```python
from build123d import *

# Parameters (mm, degrees)
SZKIC1_R                    = 7.5
SZKIC1_R_2                  = 3
DODANIE_WYCI_GNI_CIE1_DEPTH = 15
DODANIE_WYCI_GNI_CIE2_START = -15
SZKIC1_3_R                  = 7.5
SZKIC1_3_R_2                = 3
DODANIE_WYCI_GNI_CIE2_DEPTH = 15


with BuildPart() as part:
    # Szkic1 → Dodanie-wyciągnięcie1 (new body)
    # profile 1 of 2: a face of its own
    with BuildSketch(Plane(origin=(0, 0, 0), x_dir=(1, 0, 0), z_dir=(0, 1, 0))):
        Polygon((-5.484827557, -9.5), (5.484827557, -9.5), (10.969655115, 0), (5.484827557, 9.5), (-5.484827557, 9.5), (-10.969655115, 0), align=None)
        Circle(SZKIC1_R, mode=Mode.SUBTRACT)
    # profile 2 of 2: a face of its own
    with BuildSketch(Plane(origin=(0, 0, 0), x_dir=(1, 0, 0), z_dir=(0, 1, 0))):
        Circle(SZKIC1_R)
        with Locations(Location((0, 0, 0), (0, 0, 270))):
            Circle(SZKIC1_R_2, mode=Mode.SUBTRACT)
    extrude(amount=DODANIE_WYCI_GNI_CIE1_DEPTH)

    # Szkic1<3> → Dodanie-wyciągnięcie2 (add)
    with BuildSketch(Plane(origin=(0, 0, 0), x_dir=(1, 0, 0), z_dir=(0, 1, 0)).offset(DODANIE_WYCI_GNI_CIE2_START)):
        with Locations(Location((0, 0, 0), (0, 0, 270))):
            Circle(SZKIC1_3_R)
        with Locations(Location((0, 0, 0), (0, 0, 270))):
            Circle(SZKIC1_3_R_2, mode=Mode.SUBTRACT)
    extrude(amount=DODANIE_WYCI_GNI_CIE2_DEPTH)


solid = part.part
```
Can you work these out from the model? Positions are in its coordinate system, mm. A direction names the side the tool comes from. Round coordinates to 2 decimals unless told otherwise and drop trailing zeros. Loops run counter-clockwise (first coordinate to the right, second up) from the corner with the lowest first, then second, coordinate; pieces in that order, holes last.
Item 1: Suppose I cut it at C-C, the plane y = 11. Write out the boundary of the cut face in (x, z).
Item 2: Will these pins go through, and if not, where does the flat tip stop? pin 1 Ø1 at (y, z) = (-11, 5.5) entering from +X; pin 2 Ø8 at (y, z) = (-1, -5.5) entering from -X; pin 3 Ø8 at (y, z) = (-6.5, -3.5) entering from -X.
Item 3: Suppose I cut it at B-B, the plane z = -2. Write out the boundary of the cut face in (x, y), then the cut area to 3 significant figures.
Item 4: Please list where these lines run through material, in increasing order: L1, parallel to Y at x = -5.75, z = 5.5; L2, parallel to X at y = -0.25, z = 0.5; L3, parallel to X at y = -3.75, z = -1.75.
Item 5: If we mould it in two halves opening along Z, with no side actions, what happens to faces 3 (the flat face through (-8.2, 7.4, -4.8)), 4 (the flat face through (0.1, -15, 3.2)), 5 (the cylindrical face through (0.9, -0.21, 2.86)), 6 (the flat face through (8.2, 7.4, 4.8))? For each: +Z half, -Z half, draft (parallel to the pull), parting line (faces both ways), or undercut.
Item 6: Which directions (+Z, -Z, +X, -X, +Y, -Y) give clear straight access to the entire face, cutting with the end or side of a thin tool? Please do faces 1 (the flat face through (2.3, 15, -2.2)), 2 (the cylindrical face through (0.33, -7.605, -7.493)).
Item 7: Suppose I cut it at D-D, the plane x = 4.5. Write out the boundary of the cut face in (y, z).
Item 8: Suppose I cut it at A-A, the plane x = 0. Write out the boundary of the cut face in (y, z), then the cut area to 3 significant figures.
Reported:
1. outline: (-10.97, 0) - (-5.48, -9.5) - (5.48, -9.5) - (10.97, 0) - (5.48, 9.5) - (-5.48, 9.5) - close; hole circle Ø6 at (0, 0)
2. pin 1: stops at x = 5.59
2. pin 2: stops at x = -10.03
2. pin 3: stops at x = -7.5
3. outline: (-9.81, 0) - (-7.23, 0) - (-7.23, -15) - (-2.24, -15) - (-2.24, 15) - (-9.81, 15) - close; (2.24, -15) - (7.23, -15) - (7.23, 0) - (9.81, 0) - (9.81, 15) - (2.24, 15) - close
3. area: 377 mm2
4. L1: y = 0 to 15
4. L2: x = -7.48 to -2.96, 2.96 to 7.48
4. L3: x = -7.29 to -2.44, 2.44 to 7.29
5. face 3: -Z half
5. face 4: draft
5. face 5: undercut
5. face 6: +Z half
6. face 1: +Z, -Z, +X, -X, +Y
6. face 2: -Y
7. outline: (-15, -6) - (0, -6) - (0, -9.5) - (15, -9.5) - (15, 9.5) - (0, 9.5) - (0, 6) - (-15, 6) - close
8. outline: (-15, -7.5) - (0, -7.5) - (0, -9.5) - (15, -9.5) - (15, -3) - (-15, -3) - close; (-15, 3) - (15, 3) - (15, 9.5) - (0, 9.5) - (0, 7.5) - (-15, 7.5) - close
8. area: 330 mm2
